Source: CAD feature listing. Evaluate the final solid. Frame: model axes, mm. A direction names the side the tool comes from. Give positions to 0.01 mm unless a question says otherwise; leave off trailing zeros. Loops run counter-clockwise (first coordinate to the right, second up) from the corner with the lowest first, then second, coordinate; pieces in that order, holes last. Notation, with made-up numbers: M -38.5,4.5 L -18.5,4.5 A22 cw -18.5,14.5 Z; hole C 52,-14.75 d8. An arc over 180 degrees is marked long. Answer in a Markdown table with one row per item.
```python
from build123d import *

# Parameters (mm, degrees)
BOSS_EXTRUDE1_DEPTH = 50


with BuildPart() as part:
    # Sketch1 → Boss-Extrude1 (new body)
    with BuildSketch(Plane.XY):
        with BuildLine():
            Line((-0.226533162, 0), (-31.8, 0))
            Line((-31.8, 0), (-31.8, 2))
            Line((-31.8, 2), (-1.79756025, 2))
            ThreePointArc((-1.79756025, 2), (-1.552823997, 2.063990635), (-1.370731057, 2.239583333))
            ThreePointArc((-1.370731057, 2.239583333), (-0.802551257, 2.977276557), (-0.088888889, 3.575361503))
            ThreePointArc((-0.088888889, 3.575361503), (-0.023616579, 3.647376483), (0, 3.741657387))
            Line((0, 3.741657387), (0, 4))
            Line((0, 4), (2, 4))
            Line((2, 4), (2, 2.355630783))
            ThreePointArc((2, 2.355630783), (1.987179561, 2.285176459), (1.950361882, 2.223754688))
            Line((1.950361882, 2.223754688), (0.149371544, 0.170309763))
            ThreePointArc((0.149371544, 0.170309763), (-0.020190145, 0.044563331), (-0.226533162, 0))
        make_face()
    extrude(amount=-BOSS_EXTRUDE1_DEPTH)


solid = part.part
```
1) Section B-B, the plane x = -13. Return loops of the section in (y, z), then the cut area to 3 significant figures.
Reply:
| item | result |
|---|---|
| outline | M 0,-50 L 2,-50 L 2,0 L 0,0 Z |
| area | 100 mm² |
2) Section A-A, the plane z = -9.5. Return loops of the section in (x, y).
Reply:
| item | result |
|---|---|
| outline | M -31.8,0 L -0.23,0 A0.5 ccw 0.15,0.17 L 1.95,2.22 A0.2 ccw 2,2.36 L 2,4 L 0,4 L 0,3.74 A0.2 cw -0.09,3.58 A4.3 ccw -1.37,2.24 A0.5 cw -1.8,2 L -31.8,2 Z |
3) Set-up query: faces 1 (the flat face through (-17, 2, -25)), 2 (the flat face through (1, 4, -25)). Return all of +Z, -Z, +X, -X, +Y, -Y with unobstructed straight access to the full face (end or side cutting, diameter ignored); none if empty.
Reply:
| item | result |
|---|---|
| face 1 | +Z, -Z, -X, +Y |
| face 2 | +Z, -Z, +X, -X, +Y |
4) Pull-direction query (Y, two-part tool) for faces 3 (the flat face through (-31.8, 1, -25)), 4 (the cylindrical face through (-0.81, 2.97, -24.65)), 5 (the flat face through (1.06, 1.21, -24.65)); classes: released by +Y, released by -Y, zero draft, split by the parting line, or undercut.
Reply:
| item | result |
|---|---|
| face 3 | zero draft |
| face 4 | released by +Y |
| face 5 | released by -Y |
5) Section C-C, the plane y = 1.45. Return loops of the section in (x, z), then the cut area to 3 significant figures.
Reply:
| item | result |
|---|---|
| outline | M -31.8,-50 L 1.27,-50 L 1.27,0 L -31.8,0 Z |
| area | 1,650 mm² |
6) Material intervals for L1, parallel to Y at x = -12.5, z = -6; L2, parallel to X at y = 0.5, z = -44.5; L3, parallel to X at y = 1.65, z = -38.5, sorted ascending.
Reply:
| item | result |
|---|---|
| L1 | y = 0 to 2 |
| L2 | x = -31.8 to 0.44 |
| L3 | x = -31.8 to 1.45 |
7) Pin query (flat end, axial travel): pin 1 Ø6 at (x, z) = (-21.5, -43) entering from +Y; pin 2 Ø1 at (y, z) = (2, -30) entering from +X. Return the tip coordinate at first contact, or that it passes through.
Reply:
| item | result |
|---|---|
| pin 1 | stops at y = 2 |
| pin 2 | stops at x = 2 |
